Here's how the part is built. I have some questions about the finished solid (model axes, mm). A direction names the side the tool comes from. Round coordinates to 2 decimals unless told otherwise and drop trailing zeros. Loops run counter-clockwise (first coordinate to the right, second up) from the corner with the lowest first, then second, coordinate; pieces in that order, holes last. Notation, with made-up numbers: M 1,2 L 37,2 A13 ccw 37,13 Z; hole C -25.5,-34.75 d5. An arc over 180 degrees is marked long. Answer as a JSON object with one key per item and string values.
Autodesk Inventor part; units mm, degrees
ref_plane "YZ Plane" through (0, 0, 0) normal (1, 0, 0) x (0, 1, 0)
ref_plane "XZ Plane" through (0, 0, 0) normal (0, 1, 0) x (-1, 0, 0)
ref_plane "XY Plane" through (0, 0, 0) normal (0, 0, 1) x (1, 0, 0)
sketch "Sketch1" plane through (0, 0, 0) normal (0, 0, 1) x (1, 0, 0)
  circle A0 centre (0, 0) radius 2.75
  circle A1 centre (0, 0) radius 4.5
  dimension "d0" = 5.5
  dimension "d1" = 9
extrude "Extrusion1" add sketch "Sketch1" along normal blind 10
sketch "Sketch2" plane through (0, 0, 10) normal (0, 0, 1) x (1, 0, 0)
  line L0 (-10, 4.5) -> (10, 4.5)
  line L1 (10, 4.5) -> (10, -4.5)
  line L2 (10, -4.5) -> (-10, -4.5)
  line L3 (-10, -4.5) -> (-10, 4.5)
  point P0 (0, 0)
  dimension "d4" = 20
  dimension "d5" = 10
extrude "Extrusion2" add sketch "Sketch2" along normal blind 3
sketch "Sketch3" plane through (0, 0, 13) normal (0, 0, 1) x (1, 0, 0)
  line L0 (10, 4.5) -> (-10, 4.5)
  line L1 (-10, -4.5) -> (10, -4.5)
  line L2 (-10, 4.5) -> (-6, 4.5)
  line L3 (-6, 4.5) -> (-6, -4.5)
  line L4 (-6, -4.5) -> (-10, -4.5)
  line L5 (-10, -4.5) -> (-10, 4.5)
  line L6 (10.0384, 4.5) -> (6.0384, 4.5)
  line L7 (6.0384, 4.5) -> (6.0384, -4.5)
  line L8 (6.0384, -4.5) -> (10.0384, -4.5)
  line L9 (10.0384, -4.5) -> (10.0384, 4.5)
  point P0 (0, 0)
  dimension "d8" = 4
  dimension "d9" = 4
extrude "Extrusion3" add sketch "Sketch3" along normal blind 20 contours L6 L9 L8 L1 L7 L0 | L3 L1 L5 L0
sketch "Sketch4" plane through (10.0384, -4.5, 13) normal (1, 0, 0) x (0, 0, -1)
  circle A0 centre (-15, 4.5) radius 4
  point P0 (13, 4.5)
  dimension "d12" = 8
  dimension "d13" = 28
extrude "Extrusion4" cut sketch "Sketch4" against normal blind 27
properties part number "Connector"
Item 1: I want a section at A-A, the plane y = 0. State how many separate pieces and enclosed holes the cut face has, then the cut area to 3 significant figures.
Resolved:
{"separate pieces": "3", "enclosed holes": "0", "area": "191 mm²"}
Item 2: Please list where these lines run through material, in increasing order: probe 1 along X at (y, z) = (-4, 22); probe 2 along Y at (x, z) = (-7.95, 28); probe 3 along Z at (x, y) = (-2.75, 1). Write a range as from..to.
Resolved:
{"probe 1": "-10..-6, 6.04..10.04", "probe 2": "-4.5..-4, 4..4.5", "probe 3": "0..13"}
Item 3: I want a section at B-B, the plane z = 28. Please give me the cut outline in (x, y), then the cut area to 3 significant figures.
Resolved:
{"outline": "M -10,-4.5 L -6,-4.5 L -6,-4 L -10,-4 Z; M -10,4 L -6,4 L -6,4.5 L -10,4.5 Z; M 6.04,-4.5 L 10.04,-4.5 L 10.04,-4 L 6.04,-4 Z; M 6.04,4 L 10.04,4 L 10.04,4.5 L 6.04,4.5 Z", "area": "8.00 mm²"}
Item 4: I'm going to push flat-ended pins straight in: pin 1 Ø2.5 at (x, y) = (5.5, -1) entering from -Z; pin 2 Ø3.5 at (y, z) = (2, 11) entering from +X; pin 3 Ø1.6 at (x, y) = (0, 0) entering from -Z; pin 4 Ø2 at (x, z) = (4.5, 6) entering from +Y. Where does each tip first touch, or does it pass through?
Resolved:
{"pin 1": "z = 0", "pin 2": "x = 10", "pin 3": "z = 10", "pin 4": "y = 2.83"}
Item 5: If we mould it in two halves opening along X, with no side actions, what happens to faces 4 (the face through (-6, 0, 21)), 5 (the face through (8, 0, 33)), 6 (the face through (0, 0, 13)), 7 (the face through (10, 0, 11))? For each: pulls with the +X half, pulls with the -X half, needs draft (parallel to the pull), parting line crosses it, or undercut.
Resolved:
{"face 4": "undercut", "face 5": "needs draft", "face 6": "undercut", "face 7": "pulls with the +X half"}
Item 6: I want a section at D-D, the plane z = 4.5. Please give me the cut outline in (x, y), then the cut area to 3 significant figures.
Resolved:
{"outline": "C 0,0 d9; hole C 0,0 d5.5", "area": "39.9 mm²"}
Item 7: I want a section at C-C, the plane x = -7.5. Please give me the cut outline in (y, z).
Resolved:
{"outline": "M -4.5,10 L 4.5,10 L 4.5,33 L -4.5,33 Z; hole C 0,28 d8"}
Item 8: On a 3-axis mill with a long thin cutter (end or side, diameter ignored), from which of +Z, -Z, +X, -X, +Y, -Y can I reach the whole of each face in a straight line? I mean faces 1 (the face through (-0.59, -4.46, 4.93)), 2 (the face through (0, -3, 0)), 3 (the face through (6.038, 0, 21)). Say none if no direction works.
Resolved:
{"face 1": "-Z", "face 2": "-Z, +X, -X, +Y, -Y", "face 3": "+Z, +Y, -Y"}
